Input: part model. Units: mm. Frame: model coordinates. A direction names the side the tool comes from. Give positions to 0.01 mm unless a question says otherwise; leave off trailing zeros. Loops run counter-clockwise (first coordinate to the right, second up) from the corner with the lowest first, then second, coordinate; pieces in that order, holes last. Notation, with made-up numbers: M -36.75,32 L -16.75,32 A34 ccw -16.75,69 Z; hole C 20,47.5 d3. An arc over 180 degrees is marked long. Return JSON: item names as keys, results as strings. Group by question number.
```python
from build123d import *

# Parameters (mm, degrees)
SKETCH1_W                = 14
SKETCH1_H                = 9
SKETCH1_W_2              = 2
SKETCH1_H_2              = 7.2
BOSS_EXTRUDE1_DEPTH      = 1.2
BOSS_EXTRUDE2_DEPTH      = 4.5
BOSS_EXTRUDE2_DEPTH_BACK = 4.5
SKETCH2_R                = 1.75
SKETCH2_R_2              = 0.7
FILLET1_R                = 10
BOSS_EXTRUDE3_DEPTH      = 0.771345
BOSS_EXTRUDE3_DEPTH_BACK = 0.4
SKETCH3_W                = 9
SKETCH3_H                = 5
FILLET2_R                = 2


with BuildPart() as part:
    # Sketch1 → Boss-Extrude1 (new body)
    with BuildSketch(Plane(origin=(0, 0, 0), x_dir=(1, 0, 0), z_dir=(0, 1, 0))):
        Rectangle(SKETCH1_W, SKETCH1_H)
        with Locations((2.5, 0)):
            Rectangle(SKETCH1_W_2, SKETCH1_H_2, mode=Mode.SUBTRACT)
    extrude(amount=BOSS_EXTRUDE1_DEPTH)

    # Sketch2 → Boss-Extrude2 (add, two sides: drawn at the far end of the back side and taken through both)
    with BuildSketch(Plane.XY.offset(-BOSS_EXTRUDE2_DEPTH_BACK)):
        with Locations((-8.643928222, 0.6)):
            Circle(SKETCH2_R)
        with Locations((-8.643928222, 0.6)):
            Circle(SKETCH2_R_2, mode=Mode.SUBTRACT)
    extrude(amount=BOSS_EXTRUDE2_DEPTH + BOSS_EXTRUDE2_DEPTH_BACK)

    # Fillet1
    fillet1_edges = [part.edges().sort_by_distance(p)[0] for p in [
        (-7, 1.2, 0),
        (-7, 0, 0),
    ]]
    fillet(fillet1_edges, radius=FILLET1_R)

    # Sketch3 → Boss-Extrude3 (add, two sides: drawn at the far end of the back side and taken through both)
    with BuildSketch(Plane(origin=(3.51688397, -2.951016042, 0), x_dir=(0, 0, -1), z_dir=(0.7660444431189749, -0.642787609686543, 0)).offset(-BOSS_EXTRUDE3_DEPTH_BACK)):
        with Locations((0, 6.999513268)):
            Rectangle(SKETCH3_W, SKETCH3_H)
    extrude(amount=BOSS_EXTRUDE3_DEPTH + BOSS_EXTRUDE3_DEPTH_BACK)

    # Fillet2
    fillet2_edges = [part.edges().sort_by_distance(p)[0] for p in [
        (6.477837084, 1.2, 0),
    ]]
    fillet(fillet2_edges, radius=FILLET2_R)


solid = part.part
```
Item 1: Section C-C, the plane y = 0.6. Return loops of the section in (x, z), then the cut area to 3 significant figures.
Item 2: Section D-D, the plane z = 4. Return loops of the section in (x, y), then the cut area to 3 significant figures.
Item 3: Section B-B, the plane x = 3. Return loops of the section in (y, z), then the cut area to 3 significant figures.
Item 4: Material intervals for line 1 (Y direction, x = -2, z = -0.75); line 2 (X direction, y = 3.8, z = 1.5); line 3 (Y direction, x = -6.75, z = -2.5), sorted ascending. Write a range as from..to.
Item 5: First-contact query: pin 1 Ø1.1 at (x, y) = (-8.64, 0.6) entering from -Z; pin 2 Ø0.6 at (y, z) = (1, -1) entering from +X; pin 3 Ø2.5 at (x, z) = (2.5, 0.5) entering from -Y; pin 4 Ø2 at (x, z) = (-6.5, 1.5) entering from -Y. Flat tips, straight axial feed; report the tip coordinate or a pass-through.
Item 6: Pull-direction query (Y, two-part tool) for faces 6 (the face through (-1, 1, -4.5)), 7 (the face through (9.76, 4.21, 0.06)), 8 (the face through (-9.343, 0.631, -0.063)); classes: pulls with the +Y half, pulls with the -Y half, needs draft (parallel to the pull), parting line crosses it, or undercut.
Item 7: Section A-A, the plane z = 2.25. Return loops of the section in (x, y), then the cut area to 3 significant figures.
Item 8: Reachability of faces 1 (the face through (-5.76, 1.44, -0.06)), 2 (the face through (2, 1, -3.6)), 3 (the face through (-10.393, 0.649, -0.063)), 4 (the face through (0, 0, 0)), 5 (the face through (-1, 1, 4.5)) from +Z, -Z, +X, -X, +Y, -Y: full face, straight path, thin tool, end or side. Return the list, or none.
Answer below:
{
 "1": {"outline": "M -10.39,-4.5 L -9.34,-4.5 L -9.34,4.5 L -10.39,4.5 Z; M -7.94,-4.5 L 7.5,-4.5 L 7.5,4.5 L -7.94,4.5 Z; hole M 1.5,-3.6 L 3.5,-3.6 L 3.5,3.6 L 1.5,3.6 Z", "area": "134 mm^2"},
 "2": {"outline": "M -7.89,-0.98 A10 cw -3.57,0 L 7,0 L 10.21,3.83 L 9.32,4.58 L 7.08,1.91 A2 cw 5.55,1.2 L -3.57,1.2 A10 cw -7.89,2.18 A1.75 ccw long Z; hole C -8.64,0.6 d1.4", "area": "31.8 mm^2"},
 "3": {"outline": "M 0,-4.5 L 1.2,-4.5 L 1.2,-3.6 L 0,-3.6 Z; M 0,3.6 L 1.2,3.6 L 1.2,4.5 L 0,4.5 Z", "area": "2.16 mm^2"},
 "4": {"line 1": "0..1.2", "line 2": "8.66..10.19", "line 3": "-0.52..1.72"},
 "5": {"pin 1": "through", "pin 2": "x = 8.09", "pin 3": "y = 0", "pin 4": "y = -0.8"},
 "6": {"face 6": "needs draft", "face 7": "pulls with the +Y half", "face 8": "undercut"},
 "7": {"outline": "M -7.89,-0.98 A10 cw -3.57,0 L 1.5,0 L 1.5,1.2 L -3.57,1.2 A10 cw -7.89,2.18 A1.75 ccw long Z; M 3.5,0 L 7,0 L 10.21,3.83 L 9.32,4.58 L 7.08,1.91 A2 cw 5.55,1.2 L 3.5,1.2 Z; hole C -8.64,0.6 d1.4", "area": "29.4 mm^2"},
 "8": {"face 1": "+Z, -Z, +Y", "face 2": "+Y, -Y", "face 3": "+Z, -Z", "face 4": "+Z, -Z, +X, -Y", "face 5": "+Z, +X, -X, +Y, -Y"}
}
